Verification items for the finished model (mm, model axes). Give positions to 0.01 mm unless a question says otherwise; leave off trailing zeros. Order: outer loops, then holes, each group sorted by start corner. A loop starts at its lowest first (then second) coordinate and runs counter-clockwise, first axis right, second up. Notation, with made-up numbers: (67, 53) -> (73, 53) arc R13 cw to (73, 64) -> close; hole circle Ø4 at (81.25, 16.25). An arc over 180 degrees is marked (long way). Return JSON: item names as keys, results as strings. Group by question number.
(1) Cross-section at B-B on z = 0.35. State how many separate pieces and enclosed holes the cut face has, then the cut area to 3 significant figures.
(2) Cross-section at A-A on y = 38.5. Enter the section's corners in (x, z), then the cut area to 3 significant figures.
(3) Thickness scan on line 1 along X through (y, z) = (46, 1.7); line 2 along X through (y, z) = (-141.5, 0.75); line 3 along X through (y, z) = (-13, 1.55). Record the ranges inside material, lowest first.
(4) Cross-section at C-C on y = -13. Enter the section's corners in (x, z).
(5) Depth check by flat-ended pin: pin 1 Ø0.6 at (y, z) = (41, 1) entering from +X; pin 2 Ø0.6 at (y, z) = (-154.5, 0.5) entering from -X. Enter the tip coordinate at first touch or a pass-through.
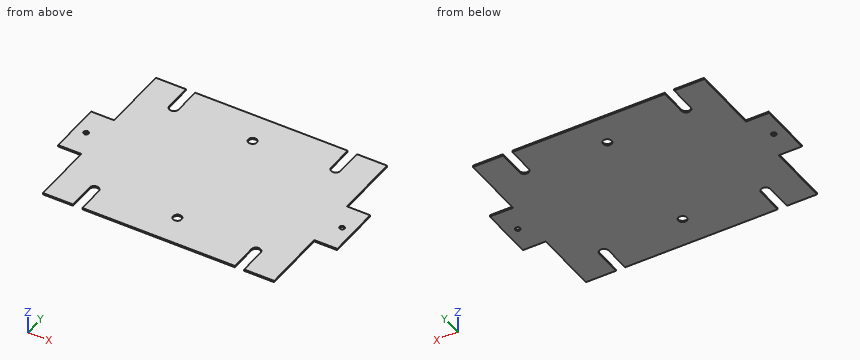
from build123d import *

# Parameters (mm, degrees)
SKETCH1_R           = 5.5
SKETCH1_R_2         = 3.25
BOSS_EXTRUDE1_DEPTH = 2


with BuildPart() as part:
    # Sketch1 → Boss-Extrude1 (new body)
    with BuildSketch(Plane.XY):
        with BuildLine():
            Line((68.948821818, -26.633764286), (98.948821818, -26.633764286))
            Line((98.948821818, -26.633764286), (98.948821818, -96.633764286))
            Line((98.948821818, -96.633764286), (68.948821818, -96.633764286))
            Line((68.948821818, -96.633764286), (68.948821818, -181.633764286))
            Line((68.948821818, -181.633764286), (29.948821818, -181.633764286))
            Line((29.948821818, -181.633764286), (29.948821818, -146.633764286))
            ThreePointArc((29.948821818, -146.633764286), (23.948821818, -140.633764286), (17.948821818, -146.633764286))
            Line((17.948821818, -146.633764286), (17.948821818, -181.633764286))
            Line((17.948821818, -181.633764286), (-180.051178182, -181.633764286))
            Line((-180.051178182, -181.633764286), (-180.051178182, -146.633764286))
            ThreePointArc((-180.051178182, -146.633764286), (-186.051178182, -140.633764286), (-192.051178182, -146.633764286))
            Line((-192.051178182, -146.633764286), (-192.051178182, -181.633764286))
            Line((-192.051178182, -181.633764286), (-231.051178182, -181.633764286))
            Line((-231.051178182, -181.633764286), (-231.051178182, -100.179856115))
            Line((-231.051178182, -100.179856115), (-261.051178182, -100.179856115))
            Line((-261.051178182, -100.179856115), (-261.051178182, -30.179856115))
            Line((-261.051178182, -30.179856115), (-231.051178182, -30.179856115))
            Line((-231.051178182, -30.179856115), (-231.051178182, 58.366235714))
            Line((-231.051178182, 58.366235714), (-192.051178182, 58.366235714))
            Line((-192.051178182, 58.366235714), (-192.051178182, 23.366235714))
            ThreePointArc((-192.051178182, 23.366235714), (-186.051178182, 17.366235714), (-180.051178182, 23.366235714))
            Line((-180.051178182, 23.366235714), (-180.051178182, 58.366235714))
            Line((-180.051178182, 58.366235714), (17.948821818, 58.366235714))
            Line((17.948821818, 58.366235714), (17.948821818, 23.366235714))
            ThreePointArc((17.948821818, 23.366235714), (23.948821818, 17.366235714), (29.948821818, 23.366235714))
            Line((29.948821818, 23.366235714), (29.948821818, 58.366235714))
            Line((29.948821818, 58.366235714), (68.948821818, 58.366235714))
            Line((68.948821818, 58.366235714), (68.948821818, -26.633764286))
        make_face()
        with Locations((-81.051178182, -141.633764286)):
            Circle(SKETCH1_R, mode=Mode.SUBTRACT)
        with Locations((-81.051178182, 18.366235714)):
            Circle(SKETCH1_R, mode=Mode.SUBTRACT)
        with Locations((83.948821818, -61.633764286)):
            Circle(SKETCH1_R_2, mode=Mode.SUBTRACT)
        with Locations((-246.051178182, -65.179856115)):
            Circle(SKETCH1_R_2, mode=Mode.SUBTRACT)
    extrude(amount=BOSS_EXTRUDE1_DEPTH)


solid = part.part
Verdict:
{
 "1": {"separate pieces": "1", "enclosed holes": "4", "area": "74,000 mm²"},
 "2": {"outline": "(-231.05, 0) -> (-192.05, 0) -> (-192.05, 2) -> (-231.05, 2) -> close; (-180.05, 0) -> (17.95, 0) -> (17.95, 2) -> (-180.05, 2) -> close; (29.95, 0) -> (68.95, 0) -> (68.95, 2) -> (29.95, 2) -> close", "area": "552 mm²"},
 "3": {"line 1": "-231.05 to -192.05, -180.05 to 17.95, 29.95 to 68.95", "line 2": "-231.05 to -189.16, -182.95 to -86.55, -75.55 to 20.84, 27.05 to 68.95", "line 3": "-231.05 to 68.95"},
 "4": {"outline": "(-231.05, 0) -> (68.95, 0) -> (68.95, 2) -> (-231.05, 2) -> close"},
 "5": {"pin 1": "x = 68.95", "pin 2": "x = -231.05"}
}
